The model under review builds one solid part; all positions refer to its coordinate system, in mm. A direction names the side the tool comes from. Round coordinates to 2 decimals unless told otherwise and drop trailing zeros. Write each loop counter-clockwise with the first axis right and the second up, starting at its lowest first coordinate (ties: lowest second). Pieces come first, ordered by that corner, then holes. Notation, with made-up numbers: M 58,6 L 78,6 A20 ccw 78,30 Z; hole C 30.25,75 d4. An arc over 180 degrees is marked long. Write item = value, one per line. Start each with the question number.
Item 1: The part is to be moulded in two halves that separate along Z. For faces 1 (the flat face through (-21, 36, 9)), 2 (the flat face through (-12, 11, -21)), 3 (the flat face through (-12, 11, 21)), say which applies: +Z half, -Z half, draft (parallel to the pull), parting line (faces both ways), or undercut.
Item 2: Tool access review of faces 4 (the flat face through (6, 12, -14)), 5 (the flat face through (0, 28, 6)), 6 (the flat face through (0, 0, 0)): name each direction out of +Z, -Z, +X, -X, +Y, -Y from which nothing blocks a thin tool from reaching the whole face with its end or side.
Item 3: For pin 1 Ø4.5 at (x, z) = (-6, -15) entering from +Y; pin 2 Ø6 at (x, y) = (-15.5, 15.5) entering from -Z; pin 3 Ø1.5 at (x, y) = (-7, 18) entering from +Z, all flat-tipped, find the tip position at first contact; note any pin that passes through.
Item 4: Take a section at C-C, the plane z = -3. Give the boundary of the cut face in (x, y), plus the area to 3 significant figures.
Item 5: To check wall thickness, follow line 1 along Z through (x, y) = (-12, 36.5); line 2 along Y through (x, z) = (-12, 9); line 3 along X through (y, z) = (32, 18.5). State the ranges of each line that lie inside material, in increasing order.
Item 6: Take a section at A-A, the plane x = 10. Give the boundary of the cut face in (y, z).
Item 7: Take a section at D-D, the plane x = -17.5. Give the boundary of the cut face in (y, z), plus the area to 3 significant figures.
Item 8: Take a section at B-B, the plane y = 5. Give the boundary of the cut face in (x, z), plus the area to 3 significant figures.
from build123d import *

# Parameters (mm, degrees)
SKETCH1_W           = 66
SKETCH1_H           = 42
BOSS_EXTRUDE1_DEPTH = 12
CHAMFER1_SIZE       = 12
CHAMFER2_SIZE       = 12
SKETCH2_W           = 54
SKETCH2_H           = 12
BOSS_EXTRUDE2_DEPTH = 42
CHAMFER3_SIZE       = 42
CHAMFER3_SIZE_2     = 55
SKETCH4_W           = 12
SKETCH4_H           = 42
BOSS_EXTRUDE3_DEPTH = 27
SKETCH7_W           = 12
SKETCH7_H           = 21
REVOLVE1_ANGLE      = 181


with BuildPart() as part:
    # Sketch1 → Boss-Extrude1 (new body)
    with BuildSketch(Plane(origin=(0, 0, 0), x_dir=(1, 0, 0), z_dir=(0, 1, 0))):
        Rectangle(SKETCH1_W, SKETCH1_H)
    extrude(amount=BOSS_EXTRUDE1_DEPTH)

    # Chamfer1
    chamfer1_edges = [part.edges().sort_by_distance(p)[0] for p in [
        (33, 6, 21),
    ]]
    chamfer(chamfer1_edges, length=CHAMFER1_SIZE)

    # Chamfer2
    chamfer2_edges = [part.edges().sort_by_distance(p)[0] for p in [
        (33, 6, -21),
    ]]
    chamfer(chamfer2_edges, length=CHAMFER2_SIZE)

    # Sketch2 → Boss-Extrude2 (add)
    with BuildSketch(Plane(origin=(0, 12, 0), x_dir=(1, 0, 0), z_dir=(0, 1, 0))):
        with Locations((6, 0)):
            Rectangle(SKETCH2_W, SKETCH2_H)
    extrude(amount=BOSS_EXTRUDE2_DEPTH)

    # Chamfer3
    # the kernel refuses this chamfer: 55, 42 mm, written as the material it takes off along each edge
    with BuildSketch(Plane(origin=(33, 54, 147.910486993), x_dir=(0.04031520079207804, -0.9991870118176548, 0), z_dir=(0, 0, -1))) as chamfer3_piece_1:
        Polygon((CHAMFER3_SIZE * 0.999187011818, CHAMFER3_SIZE * 0.0403152007921), (-CHAMFER3_SIZE_2 * 0.0403152007921, CHAMFER3_SIZE_2 * 0.999187011818), (0, 0), align=None)
    extrude(amount=295.820973986, mode=Mode.SUBTRACT)

    # Sketch4 → Boss-Extrude3 (add)
    with BuildSketch(Plane(origin=(0, 12, 0), x_dir=(1, 0, 0), z_dir=(0, 1, 0))):
        with Locations((-27, 0)):
            Rectangle(SKETCH4_W, SKETCH4_H)
    extrude(amount=BOSS_EXTRUDE3_DEPTH)

    # Sketch7 → Revolve1 (revolve)
    with BuildSketch(Plane(origin=(0, 39, 0), x_dir=(1, 0, 0), z_dir=(0, 1, 0))):
        with Locations((-27, 10.5)):
            Rectangle(SKETCH7_W, SKETCH7_H)
    revolve(axis=Axis((0, 39, 0), (1, 0, 0)), revolution_arc=REVOLVE1_ANGLE)


solid = part.part
Response values:
q1.face_1 = draft
q1.face_2 = -Z half
q1.face_3 = +Z half
q2.face_4 = -Z, +X, +Y
q2.face_5 = +Z, +X, +Y
q2.face_6 = +Z, -Z, +X, -X, -Y
q3.pin_1 = 12
q3.pin_2 = -6
q3.pin_3 = 6
q4.outline = M -33,0 L 33,0 L 33,12 L -21,53.24 L -21,59.78 L -33,59.78 Z
q4.area = 2,480 mm2
q5.line_1 = -6 to 6
q5.line_2 = 0 to 12
q5.line_3 = -33 to -21
q6.outline = M 0,-21 L 12,-21 L 12,-6 L 29.56,-6 L 29.56,6 L 12,6 L 12,21 L 0,21 Z
q7.outline = M 0,-21 L 12,-21 L 12,-6 L 50.56,-6 L 50.56,6 L 12,6 L 12,21 L 0,21 Z
q7.area = 967 mm2
q8.outline = M -33,-21 L 21,-21 L 33,-9 L 33,9 L 21,21 L -33,21 Z
q8.area = 2,630 mm2
